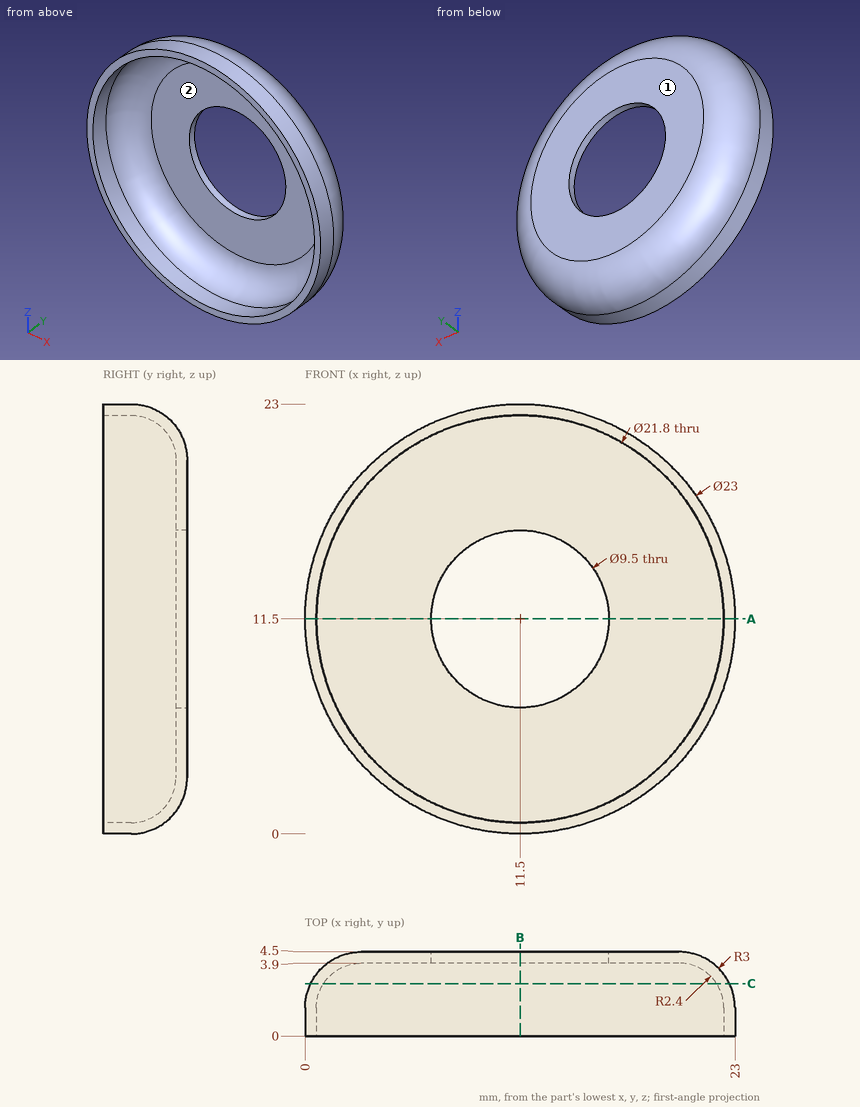
Verification items for this drawing (mm, ordinates from the low corner). Round coordinates to 2 decimals unless told otherwise and drop trailing zeros. Loops run counter-clockwise (first coordinate to the right, second up) from the corner with the lowest first, then second, coordinate; pieces in that order, holes last. Notation, with made-up numbers: M 81.5,22 L 104.5,22 A17 cw 104.5,43 Z; hole C 57,68 d11. An arc over 180 degrees is marked long. Answer as a JSON object with one key per item and string values.
1. Section check B-B (x = 11.5). Record the boundary of the cut face in (y, z), plus the area to 3 significant figures.
Reply:
{"outline": "M 0,0 L 1.5,0 A3 ccw 4.5,3 L 4.5,6.75 L 3.9,6.75 L 3.9,3 A2.4 cw 1.5,0.6 L 0,0.6 Z; M 0,22.4 L 1.5,22.4 A2.4 cw 3.9,20 L 3.9,16.25 L 4.5,16.25 L 4.5,20 A3 ccw 1.5,23 L 0,23 Z", "area": "11.4 mm²"}
2. Section check A-A (z = 11.5). Record the boundary of the cut face in (x, y), plus the area to 3 significant figures.
Reply:
{"outline": "M 0,0 L 0.6,0 L 0.6,1.5 A2.4 cw 3,3.9 L 6.75,3.9 L 6.75,4.5 L 3,4.5 A3 ccw 0,1.5 Z; M 16.25,3.9 L 20,3.9 A2.4 cw 22.4,1.5 L 22.4,0 L 23,0 L 23,1.5 A3 ccw 20,4.5 L 16.25,4.5 Z", "area": "11.4 mm²"}
3. Section check C-C (y = 2.8). Record the boundary of the cut face in (x, z).
Reply:
{"outline": "C 11.5,11.5 d22.41; hole C 11.5,11.5 d21.03"}
4. Mould release check, pull along X, two halves, no side actions. Record for the marked faces 1 and 2: pulls with the +X half, pulls with the -X half, needs draft (parallel to the pull), parting line crosses it, or undercut.
Reply:
{"face 1": "needs draft", "face 2": "undercut"}
5. Gauge pin test, flat ends, axial feed: P1, Ø4, axis at x = 10.5, z = 19, coming from the -Y side; P2, Ø5, axis at x = 14.5, z = 10.5, coming from the -Y side; P3, Ø2, axis at x = 12.5, y = 4, coming from the +Z side. Record the tip position at first contact, or that the pin passes through.
Reply:
{"P1": "stops at y = 3.65", "P2": "stops at y = 3.9", "P3": "stops at z = 22.56"}
6. Scan lines: line 1 (X direction, y = 0.5, z = 11.5); line 2 (Z direction, x = 20.75, y = 1.55); line 3 (X direction, y = 3, z = 9.5). Record each from-to range of solid material in increasing order.
Reply:
{"line 1": "x = 0 to 0.6, 22.4 to 23", "line 2": "z = 4.67 to 5.73, 17.27 to 18.33", "line 3": "x = 0.58 to 1.32, 21.68 to 22.42"}
